Design review of the part shown in the three views and the two pictorial views. Dimensions are in mm from the part's minimum x, y and z. Round coordinates to 2 decimals unless told otherwise and drop trailing zeros. Order: outer loops, then holes, each group sorted by start corner. A loop starts at its lowest first (then second) coordinate and runs counter-clockwise, first axis right, second up.
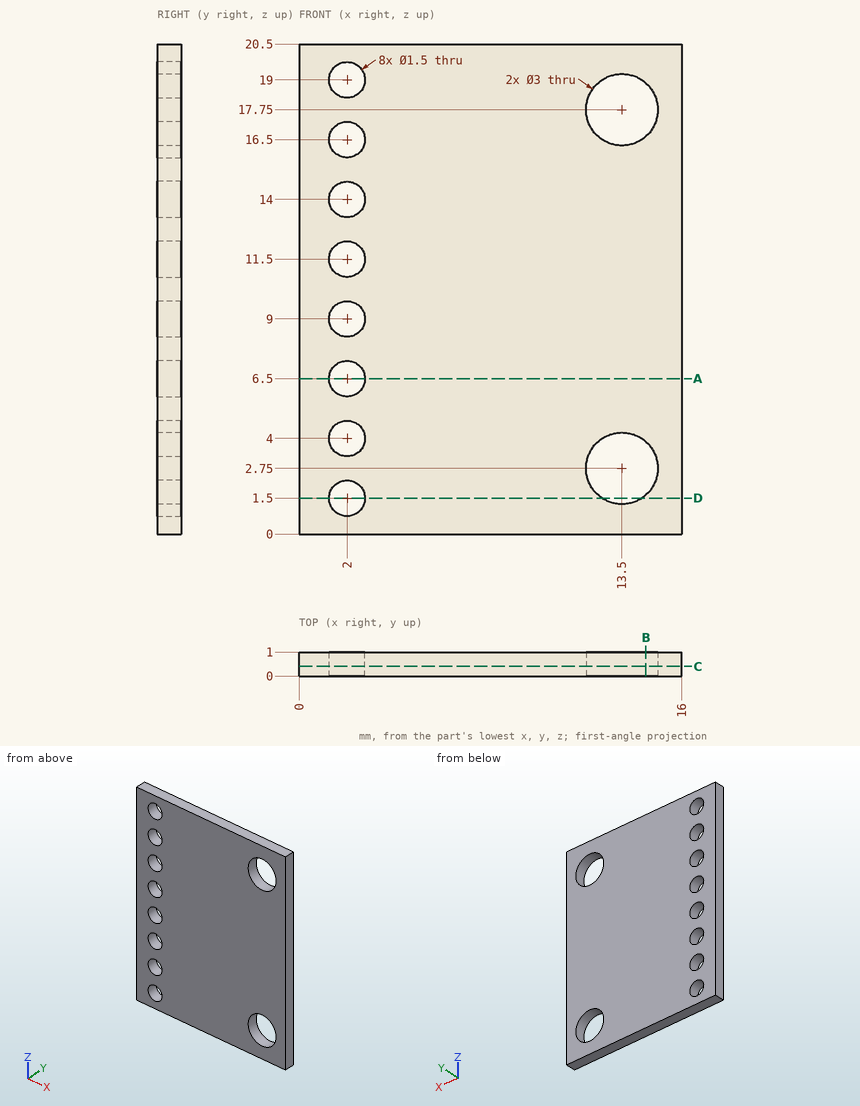
(1) Consider section C-C (y = 0.4). State how many separate pieces and enclosed holes the cut face has, and give its area (3 significant figures).
Data:
separate pieces: 1
enclosed holes: 10
area: 300 mm2
(2) Consider section A-A (z = 6.5). Write out the cut boundary in (x, y), and give its area (3 significant figures).
Data:
outline: (0, 0) - (1.25, 0) - (1.25, 1) - (0, 1) - close; (2.75, 0) - (16, 0) - (16, 1) - (2.75, 1) - close
area: 14.5 mm2
(3) Consider section D-D (z = 1.5). Write out the cut boundary in (x, y), and give its area (3 significant figures).
Data:
outline: (0, 0) - (1.25, 0) - (1.25, 1) - (0, 1) - close; (2.75, 0) - (12.67, 0) - (12.67, 1) - (2.75, 1) - close; (14.33, 0) - (16, 0) - (16, 1) - (14.33, 1) - close
area: 12.8 mm2
(4) Insertion check: pin 1 (1.4 mm diameter, centred on x = 2, z = 11.5, fed in from -Y). The pin has a flat end and moves straight along its axis. Give the tip position at first contact, or say it passes through.
Data:
pin 1: passes through
(5) To check wall thickness, follow probe 1 along X at (y, z) = (0.55, 17.75); probe 2 along X at (y, z) = (0.8, 6.5); probe 3 along X at (y, z) = (0.7, 19). State the ranges of each line that lie inside material, in increasing order.
Data:
probe 1: x = 0 to 12, 15 to 16
probe 2: x = 0 to 1.25, 2.75 to 16
probe 3: x = 0 to 1.25, 2.75 to 12.67, 14.33 to 16
(6) Consider section B-B (x = 14.5). Write out the cut boundary in (y, z), and give its area (3 significant figures).
Data:
outline: (0, 0) - (1, 0) - (1, 1.63) - (0, 1.63) - close; (0, 3.87) - (1, 3.87) - (1, 16.63) - (0, 16.63) - close; (0, 18.87) - (1, 18.87) - (1, 20.5) - (0, 20.5) - close
area: 16.0 mm2
